Design review of the part built by this model. Coordinates are the model's own, in mm. A direction names the side the tool comes from. Give positions to 0.01 mm unless a question says otherwise; leave off trailing zeros. Loops run counter-clockwise (first coordinate to the right, second up) from the corner with the lowest first, then second, coordinate; pieces in that order, holes last. Notation, with made-up numbers: (65.5, 29) - (89.5, 29) arc R18 ccw to (89.5, 40) - close; hole circle Ø5 at (21, -5.5). An arc over 180 degrees is marked (long way). Write each question's results on one line, items separated by ' | '.
Autodesk Inventor part; units mm, degrees
ref_plane "YZ Plane" through (0, 0, 0) normal (1, 0, 0) x (0, 1, 0)
ref_plane "XZ Plane" through (0, 0, 0) normal (0, 1, 0) x (-1, 0, 0)
ref_plane "XY Plane" through (0, 0, 0) normal (0, 0, 1) x (1, 0, 0)
sketch "Skizze1" plane through (0, 0, 0) normal (0, 1, 0) x (-1, 0, 0)
  line L0 (13, 0) -> (-13, 0)
  line L1 (-13, 0) -> (-13, 66)
  line L2 (-13, 66) -> (13, 66)
  line L3 (13, 66) -> (13, 0)
  point P0 (0, 0)
  point P1 (0, 0)
  dimension "d0" = 66
  dimension "d1" = 26
extrude "Extrusion1" add sketch "Skizze1" along normal blind 13
sketch "Skizze2" plane through (-13, 0, 0) normal (-1, 0, 0) x (0, 0, 1)
  line L0 (66, 0) -> (66, 13)
  line L1 (66, 6) -> (50, 6)
  line L2 (0, 13) -> (66, 13)
  line L3 (50, 6) -> (50, 0)
  line L4 (50, 0) -> (66, 0)
  line L5 (66, 6) -> (66, 0)
  point P0 (0, 0)
  dimension "d4" = 7
  dimension "d5" = 16
extrude "Extrusion2" cut sketch "Skizze2" against normal up to surface (26 mm away)
sketch "Skizze3" plane through (0, 13, 0) normal (0, 1, 0) x (1, 0, 0)
  line L0 (-13, -66) -> (13, -66)
  line L1 (13, 0) -> (-13, 0)
  point P0 (0, 0)
  point P1 (0, -58)
  point P2 (0, 0)
  dimension "d8" = 8
hole "Bohrung1" at (0, 13, 58) direction (0, -1, 0) diameter 6 depth 7 countersink diameter 12 countersink angle 90
sketch "Skizze4" plane through (0, 13, 0) normal (0, 1, 0) x (1, 0, 0)
  line L0 (13, 0) -> (-13, 0)
  point P0 (0, 0)
  point P1 (0, -8)
  point P2 (0, 0)
  point P3 (0, 0)
  dimension "d23" = 8
hole "Bohrung2" at (0, 13, 8) direction (0, -1, 0) diameter 4.134 depth 13
sketch "Skizze5" plane through (0, 13, 0) normal (0, 1, 0) x (1, 0, 0)
  line L0 (13, 0) -> (-13, 0)
  point P0 (0, 0)
  point P1 (2, -14)
  point P2 (-2, -14)
  point P3 (0, 0)
  point P4 (0, 0)
  dimension "d31" = 2
  dimension "d32" = 2
  dimension "d33" = 14
  dimension "d34" = 14
hole "Bohrung3" at (2, 13, 14) at (-2, 13, 14) direction (0, -1, 0) diameter 2 depth 13
sketch "Skizze6" plane through (-13, 0, 0) normal (-1, 0, 0) x (0, 0, 1)
  line L0 (0, 0) -> (50, 0)
  point P0 (22, 10.5)
  point P1 (22, 5)
  dimension "d42" = 22
  dimension "d43" = 5
  dimension "d44" = 5.5
hole "Bohrung4" at (-13, 5, 22) direction (1, 0, 0) diameter 4.134 depth 13 counterbore diameter 5 counterbore depth 6
hole "Bohrung5" at (-13, 10.5, 22) direction (1, 0, 0) diameter 2 depth 13
mirror "Spiegeln1" about plane through (0, 0, 0) normal (1, 0, 0) of "Bohrung4"
chamfer "Fasen1" distance 0.5 angle 45 4 edges at (-13, 13, 33) (0, 13, 66) (13, 13, 33) (0, 13, 0)
sketch "Skizze7" plane through (13, 0, 0) normal (0, 0, -1) x (-1, 0, 0)
  line L0 (0, 0) -> (0, 12.5)
  line L1 (0, 0) -> (26, 0)
  point P0 (13, 0)
  point P1 (5, 6.5)
  point P2 (21, 6.5)
  point P3 (0, 6.25)
  point P4 (0, 6.25)
  dimension "d62" = 5
  dimension "d63" = 16
  dimension "d64" = 6.5
hole "Bohrung6" at (8, 6.5, 0) at (-8, 6.5, 0) direction (0, 0, 1) diameter 4.917 depth 15
properties part number "support" material "Aluminium 6061"
(1) Take a section at A-A on z = 14. Give the boundary of the cut face in (x, y).
Answers below:
outline: (-13, 0) - (-3, 0) - (-3, 13) - (-12.5, 13) - (-13, 12.5) - close; (-1, 0) - (1, 0) - (1, 13) - (-1, 13) - close; (3, 0) - (13, 0) - (13, 12.5) - (12.5, 13) - (3, 13) - close; hole circle Ø4.92 at (-8, 6.5); hole circle Ø4.92 at (8, 6.5)
(2) Take a section at C-C on x = -8. Give the boundary of the cut face in (y, z), plus the area to 3 significant figures.
Answers below:
outline: (0, 0) - (4.04, 0) - (4.04, 15) - (8.96, 15) - (8.96, 0) - (12.5, 0) - (13, 0.5) - (13, 65.5) - (12.5, 66) - (6, 66) - (6, 50) - (0, 50) - close; hole circle Ø5 at (5, 22); hole circle Ø2 at (10.5, 22) | area: 665 mm2
(3) Tool access review of faces 1 (the cylindrical face through (-0.091, 6.409, 5.935)), 2 (the flat face through (0, 3, 50)), 3 (the flat face through (-8, 6, 15)), 4 (the flat face through (0, 10, 22)): name each direction out of +Z, -Z, +X, -X, +Y, -Y from which nothing blocks a thin tool from reaching the whole face with its end or side.
Answers below:
face 1: +Y, -Y | face 2: +Z, +X, -X, -Y | face 3: -Z | face 4: -X
(4) Take a section at D-D on x = 8. Give the boundary of the cut face in (y, z), plus the area to 3 significant figures.
Answers below:
outline: (0, 0) - (4.04, 0) - (4.04, 15) - (8.96, 15) - (8.96, 0) - (12.5, 0) - (13, 0.5) - (13, 65.5) - (12.5, 66) - (6, 66) - (6, 50) - (0, 50) - close; hole circle Ø5 at (5, 22) | area: 668 mm2
(5) Take a section at B-B on z = 22. Give the boundary of the cut face in (x, y), plus the area to 3 significant figures.
Answers below:
outline: (-13, 0) - (13, 0) - (13, 2.5) - (7, 2.5) - (7, 2.93) - (-7, 2.93) - (-7, 2.5) - (-13, 2.5) - close; (-13, 7.5) - (-7, 7.5) - (-7, 7.07) - (7, 7.07) - (7, 7.5) - (13, 7.5) - (13, 12.5) - (12.5, 13) - (-12.5, 13) - (-13, 12.5) - (-13, 11.5) - (0, 11.5) - (0, 9.5) - (-13, 9.5) - close | area: 194 mm2
(6) Wall thickness on line 1 along Y through (x, z) = (-1.25, 22); line 2 along X through (y, z) = (6.25, 8); line 3 along X through (y, z) = (6.5, 5.25): over which ranges is each line inside the solid? List them lowest first. Write a range as from..to.
Answers below:
line 1: 0..2.93, 7.07..9.5, 11.5..13 | line 2: -13..-10.45, -5.55..-2.07, 2.07..5.55, 10.45..13 | line 3: -13..-10.46, -5.54..5.54, 10.46..13
(7) Insertion check: P1, Ø1.5, axis at y = 6, z = 22.5, coming from the -X side; P2, Ø8, axis at x = 0, z = 58, coming from the -Y side; P3, Ø2.5, axis at x = -8.5, y = 7, coming from the -Z side; P4, Ø2, axis at x = 4.5, z = 58, coming from the +Y side. Each pin has a flat end and moves straight along its axis. Give the tip position at first contact, or say it passes through.
Answers below:
P1: through | P2: y = 6 | P3: z = 15 | P4: y = 12.5
(8) Draft analysis for pull direction X (two halves, no side actions). For faces 5 (the cylindrical face through (0, 8, 55)), 6 (the flat face through (0, 13, 33)), 7 (the flat face through (-13, 6, 33)), state which applies: pulls with the +X half, pulls with the -X half, needs draft (parallel to the pull), parting line crosses it, or undercut.
Answers below:
face 5: undercut | face 6: needs draft | face 7: pulls with the -X half
